Here's the drawing with two shaded views (mm, measured from the low corner). I have some questions. A direction names the side the tool comes from. Round coordinates to 2 decimals unless told otherwise and drop trailing zeros. Order: outer loops, then holes, each group sorted by start corner. A loop starts at its lowest first (then second) coordinate and runs counter-clockwise, first axis right, second up. Notation, with made-up numbers: (22, 80.5) - (73, 80.5) arc R17 cw to (73, 109.5) - close; hole circle Ø10 at (39.5, 15.25). An arc over 180 degrees is marked (long way). One line per item, written item: value.
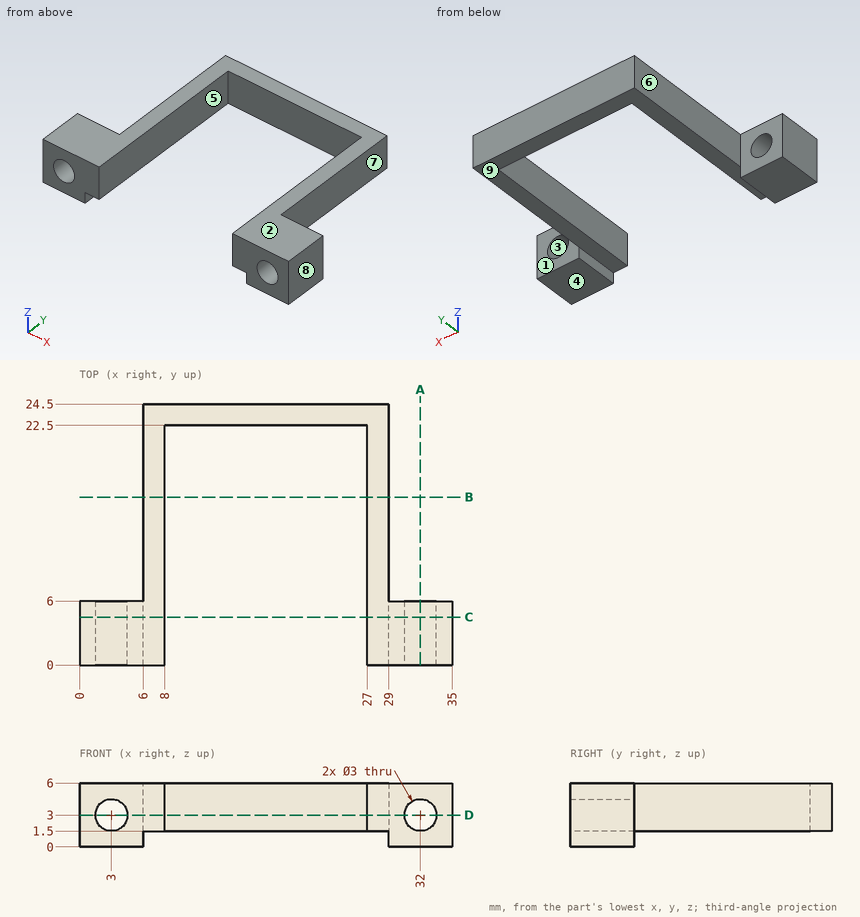
Q1. If we section it at B-B, the plane y = 15.75: Please give me the cut outline in (x, z).
Results list:
outline: (6, 1.5) - (8, 1.5) - (8, 6) - (6, 6) - close; (27, 1.5) - (29, 1.5) - (29, 6) - (27, 6) - close
Q2. If I drill on line 1 along X through (y, z) = (4, 4.65); line 2 along X through (y, z) = (5, 0.4); line 3 along X through (y, z) = (2.25, 1.95), over which ranges is the centre line in solid material (lowest first)?
Results list:
line 1: 0 to 8, 27 to 35
line 2: 0 to 6, 29 to 35
line 3: 0 to 1.93, 4.07 to 8, 27 to 30.93, 33.07 to 35
Q3. If we section it at C-C, the plane y = 4.5: Please give me the cut outline in (x, z).
Results list:
outline: (0, 0) - (6, 0) - (6, 1.5) - (8, 1.5) - (8, 6) - (0, 6) - close; (27, 1.5) - (29, 1.5) - (29, 0) - (35, 0) - (35, 6) - (27, 6) - close; hole circle Ø3 at (3, 3); hole circle Ø3 at (32, 3)
Q4. If we section it at A-A, the plane x = 32: Please give me the cut outline in (y, z).
Results list:
outline: (0, 0) - (6, 0) - (6, 1.5) - (0, 1.5) - close; (0, 4.5) - (6, 4.5) - (6, 6) - (0, 6) - close
Q5. Which directions (+Z, -Z, +X, -X, +Y, -Y) give clear straight access to the entire face, cutting with the end or side of a thin tool? Please do the marked faces 5, 6, 7, 8 and 9.
Results list:
face 5: +Z, -Z, -Y
face 6: +Z, -Z, -X, +Y
face 7: +Z, -Z, +X, +Y
face 8: +Z, -Z, +X, +Y, -Y
face 9: -Z, +Y, -Y
Q6. Will these pins go through, and if not, where does the flat tip stop? pin 1 (2 mm diameter, centred on x = 10.5, z = 1, fed in from +Y); pin 2 (3 mm diameter, centred on y = 12, z = 4, fed in from +X); pin 3 (3 mm diameter, centred on x = 33.5, z = 2.5, fed in from +Y); pin 4 (1.5 mm diameter, centred on y = 20.5, z = 5, fed in from -X).
Results list:
pin 1: y = 24.5
pin 2: x = 29
pin 3: y = 6
pin 4: x = 6
Q7. We'd pull the mould along Z, two halves only. Please class the marked faces 1, 2, 3 and 4: released by +Z, released by -Z, zero draft, split by the parting line, or undercut.
Results list:
face 1: zero draft
face 2: released by +Z
face 3: undercut
face 4: released by -Z
Q8. If we section it at D-D, the plane z = 3: Please give me the cut outline in (x, y), then the cut area to 3 significant figures.
Results list:
outline: (0, 0) - (1.5, 0) - (1.5, 6) - (0, 6) - close; (4.5, 0) - (8, 0) - (8, 22.5) - (27, 22.5) - (27, 0) - (30.5, 0) - (30.5, 6) - (29, 6) - (29, 24.5) - (6, 24.5) - (6, 6) - (4.5, 6) - close; (33.5, 0) - (35, 0) - (35, 6) - (33.5, 6) - close
area: 172 mm²
